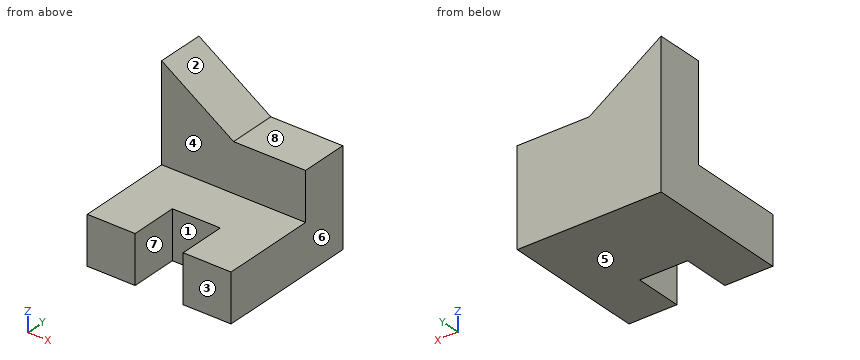
```python
from build123d import *

# Parameters (mm, degrees)
F1_DEPTH = 15
F4_DEPTH = 10.001
F3_W     = 10
F3_H     = 10
F5_DEPTH = 10.001


with BuildPart() as f1:
    # F0 (on Right) → F1 (new body, symmetric)
    with BuildSketch(Plane.YZ):
        Polygon((0, 10), (0, 0), (30, 0), (30, 30), (20, 30), (20, 10), align=None)
    extrude(amount=F1_DEPTH, both=True)

    # F2 (on face) → F4 (cut, through all)
    with BuildSketch(Plane.XZ.offset(-20)):
        Polygon((15, 30), (-15, 30), (0, 20), (15, 20), align=None)
    extrude(amount=-F4_DEPTH, mode=Mode.SUBTRACT)

    # F3 (on face) → F5 (cut, through all)
    with BuildSketch(Plane.XY.offset(10)):
        with Locations((0, 5)):
            Rectangle(F3_W, F3_H)
    extrude(amount=-F5_DEPTH, mode=Mode.SUBTRACT)


solid = f1.part
```
Here's how the part is built. I have some questions about the finished solid (model axes, mm). Face numbers are marked on the shaded views. A direction names the side the tool comes from. Round coordinates to 2 decimals unless told otherwise and drop trailing zeros. Write each loop counter-clockwise with the first axis right and the second up, starting at its lowest first coordinate (ties: lowest second). Pieces come first, ordered by that corner, then holes.
Q1. Which directions (+Z, -Z, +X, -X, +Y, -Y) give clear straight access to the entire face, cutting with the end or side of a thin tool? Please do the marked faces 4, 5, 6, 7 and 8.
Q2. If we section it at A-A on z = 5: Write out the boundary of the cut face in (x, y).
Q3. If we section it at D-D on z = 24: Write out the boundary of the cut face in (x, y).
Q4. If we mould it in two halves opening along X, with no side actions, what happens to the marked faces 1, 2 and 3? For each: +X half, -X half, draft (parallel to the pull), parting line (faces both ways), or undercut.
Q5. If we section it at B-B on y = 22.5: Write out the boundary of the cut face in (x, z).
Q6. Will these pins go through, and if not, where does the flat tip stop? P1, Ø1.5, axis at x = 1.5, z = 14.5, coming from the -Y side; P2, Ø10, axis at x = -9.5, y = 4.5, coming from the +Z side; P3, Ø5, axis at x = 6.5, y = 23.5, coming from the +Z side.
Q7. If we section it at C-C on x = 3.75: Write out the boundary of the cut face in (y, z), plus the area to 3 significant figures.
Q8. Please list where these lines run through material, in increasing order: probe 1 along X at (y, z) = (9, 9); probe 2 along Z at (x, y) = (2.75, 17.75); probe 3 along Z at (x, y) = (11, 22).
Answer below:
1. face 4: +Z, +X, -X, -Y
1. face 5: -Z, +X, -X, +Y, -Y
1. face 6: +Z, -Z, +X, +Y, -Y
1. face 7: +Z, -Z, -Y
1. face 8: +Z, +X, +Y, -Y
2. outline: (-15, 0) - (-5, 0) - (-5, 10) - (5, 10) - (5, 0) - (15, 0) - (15, 30) - (-15, 30) - close
3. outline: (-15, 20) - (-6, 20) - (-6, 30) - (-15, 30) - close
4. face 1: undercut
4. face 2: +X half
4. face 3: draft
5. outline: (-15, 0) - (15, 0) - (15, 20) - (0, 20) - (-15, 30) - close
6. P1: stops at y = 20
6. P2: stops at z = 10
6. P3: stops at z = 20
7. outline: (10, 0) - (30, 0) - (30, 20) - (20, 20) - (20, 10) - (10, 10) - close
7. area: 300 mm2
8. probe 1: x = -15 to -5, 5 to 15
8. probe 2: z = 0 to 10
8. probe 3: z = 0 to 20
